Geometry check sheet. Reference: the model listing, model coordinates, mm. Face numbers are marked on the shaded views. A direction names the side the tool comes from. Coordinates: 2 decimals unless noted, no trailing zeros. Loops run counter-clockwise (first coordinate to the right, second up) from the corner with the lowest first, then second, coordinate; pieces in that order, holes last. Notation, with made-up numbers: (49.5, 55) - (96.5, 55) arc R12 cw to (96.5, 67) - close; hole circle Ø11 at (-7, 70.5). An arc over 180 degrees is marked (long way). One line per item, written item: value.
from build123d import *

# Parameters (mm, degrees)
BOSS_EXTRUDE1_DEPTH       = 10
BOSS_EXTRUDE2_DEPTH       = 170
BOSS_EXTRUDE3_REACH       = 182
BOSS_EXTRUDE4_REACH       = 102
SKETCH8_W                 = 170
SKETCH8_H                 = 9.5
SKETCH9_W                 = 31
SKETCH9_H                 = 19.5
CUT_EXTRUDE1_DEPTH        = 10
SKETCH10_R                = 2.1
CUT_EXTRUDE2_DEPTH        = 20
F_4_0MM_DOWEL_HOLE1_D     = 4.2
F_4_0MM_DOWEL_HOLE1_DEPTH = 10
F_4_0MM_DOWEL_HOLE1_TIP   = 1.2618073
SKETCH13_R                = 2.1
CUT_EXTRUDE3_DEPTH        = 10
BOSS_EXTRUDE5_DEPTH       = 10
CUT_EXTRUDE4_REACH        = 182
SKETCH15_R                = 1.6


with BuildPart() as part:
    # Sketch5 → Boss-Extrude1 (new body)
    with BuildSketch(Plane(origin=(0, 0, 0), x_dir=(0, 0, -1), z_dir=(1, 0, 0))):
        Polygon((0, 0), (10, 90), (100, 100), (100, -100), (10, -90), align=None)
    extrude(amount=-BOSS_EXTRUDE1_DEPTH)

    # Sketch6 → Boss-Extrude2 (add)
    with BuildSketch(Plane(origin=(0, 0, 0), x_dir=(0, 0, -1), z_dir=(1, 0, 0))):
        Polygon((0, 0), (10, -90), (100, -100), (100, -90), (19, -81), (10, 0), (19, 81), (100, 90), (100, 100), (10, 90), align=None)
    extrude(amount=BOSS_EXTRUDE2_DEPTH)

    # Sketch7 → Boss-Extrude3 (add, up to next)
    with BuildSketch(Plane(origin=(170, 0, 0), x_dir=(0, 0, -1), z_dir=(1, 0, 0)), mode=Mode.PRIVATE) as boss_extrude3_sk1:
        Polygon((19, 81), (10, 0), (19, -81), (33.5, -82.611111111), (33.5, 82.611111111), align=None)
    boss_extrude3_tool1 = extrude(boss_extrude3_sk1.sketch, amount=-BOSS_EXTRUDE3_REACH, mode=Mode.PRIVATE) - part.part
    add(boss_extrude3_tool1.solids().sort_by_distance((170, 0, -23.858858))[0])

    # Sketch8 → Boss-Extrude4 (add, up to next)
    with BuildSketch(Plane(origin=(0, 0, -100), x_dir=(-1, 0, 0), z_dir=(0, 0, -1)), mode=Mode.PRIVATE) as boss_extrude4_sk1:
        with Locations((-85, 85.25)):
            Rectangle(SKETCH8_W, SKETCH8_H)
    boss_extrude4_tool1 = extrude(boss_extrude4_sk1.sketch, amount=-BOSS_EXTRUDE4_REACH, mode=Mode.PRIVATE) - part.part
    add(boss_extrude4_tool1.solids().sort_by_distance((85, 85.25, -100))[0])
    # Sketch8 → Boss-Extrude4 (add, up to next)
    with BuildSketch(Plane(origin=(0, 0, -100), x_dir=(-1, 0, 0), z_dir=(0, 0, -1)), mode=Mode.PRIVATE) as boss_extrude4_sk2:
        with Locations((-85, -85.25)):
            Rectangle(SKETCH8_W, SKETCH8_H)
    boss_extrude4_tool2 = extrude(boss_extrude4_sk2.sketch, amount=-BOSS_EXTRUDE4_REACH, mode=Mode.PRIVATE) - part.part
    add(boss_extrude4_tool2.solids().sort_by_distance((85, -85.25, -100))[0])

    # Sketch9 → Cut-Extrude1 (cut)
    with BuildSketch(Plane(origin=(0, 0, -100), x_dir=(-1, 0, 0), z_dir=(0, 0, -1))):
        with Locations((-29, -90.25)):
            Rectangle(SKETCH9_W, SKETCH9_H)
        with Locations((-29, 90.25)):
            Rectangle(SKETCH9_W, SKETCH9_H)
    extrude(amount=-CUT_EXTRUDE1_DEPTH, mode=Mode.SUBTRACT)

    # Sketch10 → Cut-Extrude2 (cut)
    with BuildSketch(Plane(origin=(0, 0, -100), x_dir=(-1, 0, 0), z_dir=(0, 0, -1))):
        with Locations((-22, -90.25)):
            Circle(SKETCH10_R)
        with Locations((-22, 90.25)):
            Circle(SKETCH10_R)
        with Locations((-36, -90.25)):
            Circle(SKETCH10_R)
        with Locations((-36, 90.25)):
            Circle(SKETCH10_R)
    extrude(amount=-CUT_EXTRUDE2_DEPTH, mode=Mode.SUBTRACT)

    # Ø4.0mm Dowel Hole1
    with Locations(Plane(origin=(0, 0, -100), x_dir=(-1, 0, 0), z_dir=(0, 0, -1))):
        with Locations((-157.5, 90.25), (-137.5, 90.25), (-117.5, 90.25), (-97.5, 90.25), (-77.5, 90.25), (-57.5, 90.25), (-157.5, -90.25), (-137.5, -90.25), (-117.5, -90.25), (-97.5, -90.25), (-77.5, -90.25), (-57.5, -90.25)):
            Hole(F_4_0MM_DOWEL_HOLE1_D / 2, depth=F_4_0MM_DOWEL_HOLE1_DEPTH)
            with Locations((0, 0, -(F_4_0MM_DOWEL_HOLE1_DEPTH + F_4_0MM_DOWEL_HOLE1_TIP / 2))):  # 118° drill point
                Cone(0, F_4_0MM_DOWEL_HOLE1_D / 2, F_4_0MM_DOWEL_HOLE1_TIP, mode=Mode.SUBTRACT)

    # Sketch13 → Cut-Extrude3 (cut)
    with BuildSketch(Plane(origin=(0, 0, 0), x_dir=(1, 0, 0), z_dir=(0, -0.110431526, 0.993883735))):
        with Locations((3.75, -31.944444444)):
            Circle(SKETCH13_R)
        with Locations((51.25, -31.944444444)):
            Circle(SKETCH13_R)
        with Locations((3.75, -71.944444444)):
            Circle(SKETCH13_R)
        with Locations((51.25, -71.944444444)):
            Circle(SKETCH13_R)
        with Locations((158.75, -31.888888889)):
            Circle(SKETCH13_R)
        with Locations((158.75, -71.888888889)):
            Circle(SKETCH13_R)
    cut_extrude3 = extrude(amount=-CUT_EXTRUDE3_DEPTH, mode=Mode.SUBTRACT)

    # Mirror1: Cut-Extrude3 across plane
    add(cut_extrude3.mirror(Plane.ZX), mode=Mode.SUBTRACT)

    # Sketch14 → Boss-Extrude5 (add)
    with BuildSketch(Plane(origin=(170, 0, 0), x_dir=(0, 0, -1), z_dir=(1, 0, 0))):
        Polygon((60, 95.555555556), (100, 100), (100, 112.5), (60, 112.5), align=None)
        Polygon((100, -100), (100, -112.5), (60, -112.5), (60, -95.555555556), align=None)
    extrude(amount=-BOSS_EXTRUDE5_DEPTH)

    # Sketch15 → Cut-Extrude4 (cut, up to next)
    with BuildSketch(Plane(origin=(170, 0, 0), x_dir=(0, 0, -1), z_dir=(1, 0, 0)), mode=Mode.PRIVATE) as cut_extrude4_sk1:
        with Locations((70, -105)):
            Circle(SKETCH15_R)
    cut_extrude4_tool1 = extrude(cut_extrude4_sk1.sketch, amount=-CUT_EXTRUDE4_REACH, mode=Mode.PRIVATE) & part.part
    add(cut_extrude4_tool1.solids().sort_by_distance((170, -105, -70))[0], mode=Mode.SUBTRACT)
    # Sketch15 → Cut-Extrude4 (cut, up to next)
    with BuildSketch(Plane(origin=(170, 0, 0), x_dir=(0, 0, -1), z_dir=(1, 0, 0)), mode=Mode.PRIVATE) as cut_extrude4_sk2:
        with Locations((90, -105)):
            Circle(SKETCH15_R)
    cut_extrude4_tool2 = extrude(cut_extrude4_sk2.sketch, amount=-CUT_EXTRUDE4_REACH, mode=Mode.PRIVATE) & part.part
    add(cut_extrude4_tool2.solids().sort_by_distance((170, -105, -90))[0], mode=Mode.SUBTRACT)
    # Sketch15 → Cut-Extrude4 (cut, up to next)
    with BuildSketch(Plane(origin=(170, 0, 0), x_dir=(0, 0, -1), z_dir=(1, 0, 0)), mode=Mode.PRIVATE) as cut_extrude4_sk3:
        with Locations((90, 105)):
            Circle(SKETCH15_R)
    cut_extrude4_tool3 = extrude(cut_extrude4_sk3.sketch, amount=-CUT_EXTRUDE4_REACH, mode=Mode.PRIVATE) & part.part
    add(cut_extrude4_tool3.solids().sort_by_distance((170, 105, -90))[0], mode=Mode.SUBTRACT)
    # Sketch15 → Cut-Extrude4 (cut, up to next)
    with BuildSketch(Plane(origin=(170, 0, 0), x_dir=(0, 0, -1), z_dir=(1, 0, 0)), mode=Mode.PRIVATE) as cut_extrude4_sk4:
        with Locations((70, 105)):
            Circle(SKETCH15_R)
    cut_extrude4_tool4 = extrude(cut_extrude4_sk4.sketch, amount=-CUT_EXTRUDE4_REACH, mode=Mode.PRIVATE) & part.part
    add(cut_extrude4_tool4.solids().sort_by_distance((170, 105, -70))[0], mode=Mode.SUBTRACT)


solid = part.part
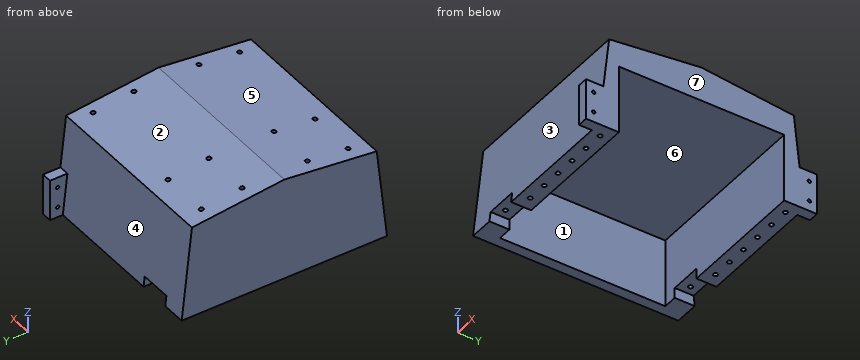
(1) Cross-section at C-C on z = -29. Record the cut outline in (x, y), and give its area (3 significant figures).
Reply:
outline: (-10, -92.11) - (170, -92.11) - (170, 92.11) - (-10, 92.11) - close
area: 33,200 mm2
(2) Cross-section at B-B on x = 130. Record the cut outline in (y, z).
Reply:
outline: (-100, -100) - (-80.5, -100) - (-80.5, -33.5) - (80.5, -33.5) - (80.5, -100) - (100, -100) - (90, -10) - (0, 0) - (-90, -10) - close
(3) Access from +Z, -Z, +X, -X, +Y, -Y to the whole of each face (thin tool, end or side, straight path). Record for the marked faces 1, 2 and 3.
Reply:
face 1: -Z, +X
face 2: +Z, +X, -X, +Y
face 3: +Z, -X, -Y
(4) Release check for a two-part mould opening along Y. For the marked faces 4, 5, 6 and 7 record: pulls with the +Y half, pulls with the -Y half, needs draft (parallel to the pull), parting line crosses it, or undercut.
Reply:
face 4: pulls with the +Y half
face 5: pulls with the -Y half
face 6: undercut
face 7: needs draft
(5) Material ranges on probe 1 along Y at (x, z) = (168, -70); probe 2 along X at (y, z) = (-22, -67); probe 3 along Y at (x, z) = (151.5, -31), recorded low to high. Write a range as from..to.
Reply:
probe 1: -112.5..-106.6, -103.4..-80.5, 80.5..103.4, 106.6..112.5
probe 2: -10..0
probe 3: -92.33..92.33
(6) Go/stop test with flat-tipped pins: pin 1 Ø3 at (x, z) = (46, -20) entering from +Y; pin 2 Ø3 at (x, y) = (164, 103) entering from +Z; pin 3 Ø3.5 at (x, y) = (36, 91) entering from -Z; pin 4 Ø1.9 at (y, z) = (-105, -90) entering from +X. Record where each tip stops, or that it passes through.
Reply:
pin 1: y = 91.28
pin 2: z = -60
pin 3: z = -90
pin 4: through
(7) Cross-section at A-A on x = 41.5. Record the cut outline in (y, z).
Reply:
outline: (-98.89, -90) - (-80.5, -90) - (-80.5, -33.5) - (80.5, -33.5) - (80.5, -90) - (98.89, -90) - (90, -10) - (0, 0) - (-90, -10) - close
